```python
from build123d import *

# Parameters (mm, degrees)
F1_DEPTH = 4
F2_DEPTH = 6


# Not quite as in the source:
# - the program builds the solid bodies; features that only make, move or delete a surface that nothing else refers to are left out


with BuildPart() as f1:
    # F0 (on Top) → F1 (new body)
    with BuildSketch(Plane.XY):
        Polygon((21.7038933188, 40.663164109), (8.2595115528, 36.550603807), (7.4202134274, 34.8720103502), (16.652489081, 23.793278262), (15.8971212804, 8.1823393703), (16.652489081, 7.4269715697), (29.9416775716, 14.0020314224), (43.0064387619, 7.4269715697), (44.5331511124, 8.1823393703), (43.0064387619, 23.793278262), (52.1547831595, 34.8720103502), (51.3386978339, 36.5214419841), (38.3063703775, 40.663164109), (31.5554067492, 51.5035130084), (30.5740684422, 53.0792954037), (29.1223078966, 53.0792954037), align=None)
        with BuildLine():
            add(Edge.make_bspline(
                [(25.3811851144, 37.6416891813), (24.5993217345, 37.4863257412), (22.5300561127, 34.3153306276), (22.8365480412, 25.5837934463), (27.8864125101, 25.4534071145), (27.6429800893, 36.1332272512), (25.9635847642, 37.7574173449), (25.3811851144, 37.6416891813)],
                knots=[0, 0, 0, 0, 0.1813668972, 0.4393300523, 0.5815805793, 0.8649022066, 1, 1, 1, 1], degree=3))
        make_face(mode=Mode.SUBTRACT)
        with BuildLine():
            add(Edge.make_bspline(
                [(34.3616716564, 37.2220426798), (33.4467151003, 37.7104749668), (31.1715810093, 33.5652339009), (32.5688269727, 27.7274369068), (33.6539912936, 25.4758331021), (37.7493894328, 26.2185759497), (35.846752744, 36.4292601731), (34.3616716564, 37.2220426798)],
                knots=[0, 0, 0, 0, 0.1841149483, 0.4213807172, 0.554620993, 0.7011599886, 1, 1, 1, 1], degree=3))
        make_face(mode=Mode.SUBTRACT)
    extrude(amount=F1_DEPTH)

    # F0 (on Top) → F2 (join)
    with BuildSketch(Plane.XY):
        Polygon((27.1650796672, 56.0378708923), (19.8419597, 43.2266667485), (5.7267113589, 38.7097857893), (4.3151844293, 35.039819777), (14.0547072515, 23.1830105186), (12.6431845129, 8.5031520575), (14.3370144069, 4.974339623), (17.900740458, 4.6316741696), (30.0049390644, 10.6204394251), (42.1440564096, 4.974339623), (45.7077824607, 4.6316741696), (47.5078485906, 8.5031520575), (45.7077824607, 22.7595549077), (55.9770017862, 34.4752110541), (54.1420131922, 39.5567007363), (39.7444628179, 43.9324304461), (32.6868370175, 55.5069334805), align=None)
        Polygon((7.4202134274, 34.8720103502), (8.2595115528, 36.550603807), (21.7038933188, 40.663164109), (29.1223078966, 53.0792954037), (30.5740684422, 53.0792954037), (31.5554067492, 51.5035130084), (38.3063703775, 40.663164109), (51.3386978339, 36.5214419841), (52.1547831595, 34.8720103502), (43.0064387619, 23.793278262), (44.5331511124, 8.1823393703), (43.0064387619, 7.4269715697), (29.9416775716, 14.0020314224), (16.652489081, 7.4269715697), (15.8971212804, 8.1823393703), (16.652489081, 23.793278262), align=None, mode=Mode.SUBTRACT)
    extrude(amount=F2_DEPTH)


solid = f1.part
```
Geometry check sheet. Reference: the model listing, model coordinates, mm. A direction names the side the tool comes from. Give positions to 0.01 mm unless a question says otherwise; leave off trailing zeros. Order: outer loops, then holes, each group sorted by start corner. A loop starts at its lowest first (then second) coordinate and runs counter-clockwise, first axis right, second up.
1. Section check A-A, the plane x = 28.5. Enter the section's corners in (y, z), and give its area (3 significant figures).
2. Section check C-C, the plane z = 3. Give the number of separate pieces and of enclosed holes in the cut face, and give its area (3 significant figures).
3. Gauge pin test, flat ends, axial feed: pin 1 Ø1 at (y, z) = (45.5, 4) entering from -X; pin 2 Ø1 at (y, z) = (38.5, 5) entering from +X; pin 3 Ø2 at (x, y) = (27, 23) entering from +Z. Record the tip position at first contact, or that the pin passes through.
4. Thickness scan on L1, parallel to X at y = 27, z = 3; L2, parallel to X at y = 35, z = 0.5; L3, parallel to Z at x = 32, y = 18.5. Record the ranges inside material, lowest first.
5. Access from +Z, -Z, +X, -X, +Y, -Y to the whole of each face (thin tool, end or side, straight path). Record for faces 1 (the face through (47.044, 41.714, 2.958)), 2 (the face through (43.76, 16.1, 4.99)), 3 (the face through (43.901, 4.805, 2.958)), 4 (the face through (12.88, 41, 2.96)), 5 (the face through (13.36, 15.95, 2.96)).
6. Section check B-B, the plane y = 46.5. Enter the section's corners in (x, z).
Values follow:
1. outline: (9.88, 0) - (55.91, 0) - (55.91, 6) - (52.04, 6) - (52.04, 4) - (13.29, 4) - (13.29, 6) - (9.88, 6) - close
1. area: 199 mm2
2. separate pieces: 1
2. enclosed holes: 2
2. area: 1,470 mm2
3. pin 1: stops at x = 20.86
3. pin 2: stops at x = 54.7
3. pin 3: stops at z = 4
4. L1: x = 10.92 to 23.59, 26.82 to 32.98, 36.1 to 49.42
4. L2: x = 4.35 to 23.48, 27.16 to 32.34, 35.64 to 55.79
4. L3: z = 0 to 4
5. face 1: +Z, -Z, +X, +Y
5. face 2: +Z
5. face 3: +Z, -Z, -Y
5. face 4: +Z, -Z, -X, +Y
5. face 5: +Z, -Z, -X
6. outline: (21.71, 0) - (38.18, 0) - (38.18, 6) - (34.67, 6) - (34.67, 4) - (25.19, 4) - (25.19, 6) - (21.71, 6) - close
